from build123d import *

# Parameters (mm, degrees)
F0_R     = 11.25
F1_DEPTH = 7


with BuildPart() as f1:
    # F0 (on Top) → F1 (new body)
    with BuildSketch(Plane.XY):
        with BuildLine():
            ThreePointArc((8.660254, -13.75), (16.25, 0), (8.660254, 13.75))
            ThreePointArc((8.660254, 13.75), (0, 43.75), (-8.660254, 13.75))
            ThreePointArc((-8.660254, 13.75), (-16.25, 0), (-8.660254, -13.75))
            ThreePointArc((-8.660254, -13.75), (0, -43.75), (8.660254, -13.75))
        make_face()
        with Locations((0, -27.5)):
            Circle(F0_R, mode=Mode.SUBTRACT)
        Circle(F0_R, mode=Mode.SUBTRACT)
        with Locations((0, 27.5)):
            Circle(F0_R, mode=Mode.SUBTRACT)
    extrude(amount=F1_DEPTH)


solid = f1.part
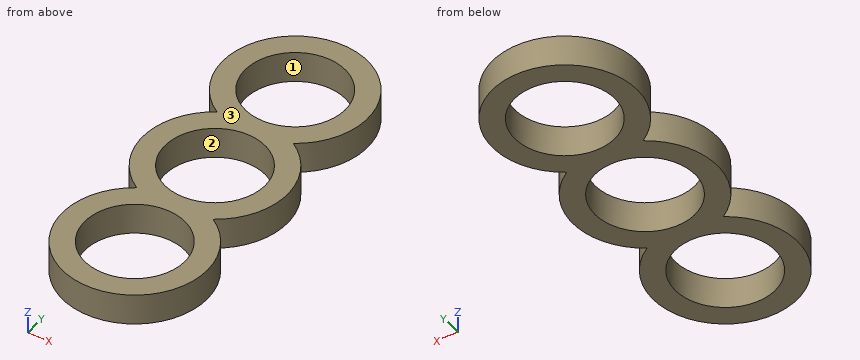
Part model, mm, in its own coordinate system. Face numbers are marked on the shaded views. Give positions to 0.01 mm unless a question says otherwise; leave off trailing zeros. Order: outer loops, then holes, each group sorted by start corner. A loop starts at its lowest first (then second) coordinate and runs counter-clockwise, first axis right, second up. Notation, with made-up numbers: (2.5, 59.25) - (35.5, 59.25) arc R24 ccw to (35.5, 88.25) - close; hole circle Ø10 at (-1, 9). An arc over 180 degrees is marked (long way). One line per question, with ' | ' between items.
1. Band-saw the part on B-B on z = 1.5. List the corners of the cut face in (x, y), then the cut area to 3 significant figures.
Filled in:
outline: (-8.66, -13.75) arc R16.25 ccw (long way) to (8.66, -13.75) arc R16.25 ccw to (8.66, 13.75) arc R16.25 ccw (long way) to (-8.66, 13.75) arc R16.25 ccw to start; hole circle Ø22.5 at (0, -27.5); hole circle Ø22.5 at (0, 0); hole circle Ø22.5 at (0, 27.5) | area: 1,180 mm²
2. Band-saw the part on D-D on x = 12.5. List the corners of the cut face in (y, z).
Filled in:
outline: (-37.88, 0) - (-17.12, 0) - (-17.12, 7) - (-37.88, 7) - close; (-10.38, 0) - (10.38, 0) - (10.38, 7) - (-10.38, 7) - close; (17.12, 0) - (37.88, 0) - (37.88, 7) - (17.12, 7) - close
3. Band-saw the part on A-A on x = 0. List the corners of the cut face in (y, z), then the cut area to 3 significant figures.
Filled in:
outline: (-43.75, 0) - (-38.75, 0) - (-38.75, 7) - (-43.75, 7) - close; (-16.25, 0) - (-11.25, 0) - (-11.25, 7) - (-16.25, 7) - close; (11.25, 0) - (16.25, 0) - (16.25, 7) - (11.25, 7) - close; (38.75, 0) - (43.75, 0) - (43.75, 7) - (38.75, 7) - close | area: 140 mm²
4. Pull direction X, two halves, no side cores. Call the marked faces 1, 2 and 3: +X half, -X half, draft (parallel to the pull), parting line (faces both ways), or undercut.
Filled in:
face 1: undercut | face 2: undercut | face 3: draft
5. Drill centre lines: probe 1 along Y at (x, z) = (13, 5.25); probe 2 along X at (y, z) = (27, 5); probe 3 along Y at (x, z) = (11.5, 5). Where is each one in solid material? Low to high.
Filled in:
probe 1: -37.25 to -17.75, -9.75 to 9.75, 17.75 to 37.25 | probe 2: -16.24 to -11.24, 11.24 to 16.24 | probe 3: -38.98 to -16.02, -11.48 to 11.48, 16.02 to 38.98
6. Drop flat-ended pins along their axis: P1, Ø8, axis at x = 7, y = -35, coming from the -Z side; P2, Ø1, axis at y = 20, z = 1.5, coming from the -X side (3 decimals); P3, Ø2, axis at y = -25, z = 4.5, coming from the +X side; P4, Ø3, axis at y = 6, z = 1.5, coming from the -X side. Give the stop position or say it passes through.
Filled in:
P1: z = 0 | P2: x = -14.665 | P3: x = 16.18 | P4: x = -15.61
7. Band-saw the part on C-C on y = 0. List the corners of the cut face in (x, z).
Filled in:
outline: (-16.25, 0) - (-11.25, 0) - (-11.25, 7) - (-16.25, 7) - close; (11.25, 0) - (16.25, 0) - (16.25, 7) - (11.25, 7) - close
